Part model, mm, in its own coordinate system. Coordinates: 2 decimals unless noted, no trailing zeros. Loops run counter-clockwise (first coordinate to the right, second up) from the corner with the lowest first, then second, coordinate; pieces in that order, holes last. Notation, with made-up numbers: (-37, 30) - (3, 30) arc R28 cw to (3, 50) - close; hole circle Ø7 at (29.5, -26.5). An arc over 180 degrees is marked (long way). Answer as CSV lines item,"result".
from build123d import *

# Parameters (mm, degrees)
SKETCH_1_R                  = 17.5
SKETCH_1_R_2                = 11
EXTRUDE_1_DEPTH             = 2
HOLE_WIZARD_M3_1_AT_2_COUNT = 2
HOLE_WIZARD_M3_1_AT_2_PITCH = 20.152543264
HOLE_WIZARD_M3_1_AT_3_COUNT = 2
HOLE_WIZARD_M3_1_AT_3_PITCH = 28.5
HOLE_WIZARD_M3_1_AT_4_COUNT = 2
HOLE_WIZARD_M3_1_AT_4_PITCH = 20.152543264
HOLE_WIZARD_M3_1_AT_5_COUNT = 2
HOLE_WIZARD_M3_1_AT_5_PITCH = 14.25
CHAMFER_1_SIZE              = 0.25


with BuildPart() as part:
    # ｽｹｯﾁ1 → ﾎﾞｽ - 押し出し1 (new body)
    with BuildSketch(Plane.XY):
        Circle(SKETCH_1_R)
        Circle(SKETCH_1_R_2, mode=Mode.SUBTRACT)
    extrude(amount=EXTRUDE_1_DEPTH)

    # ｽｹｯﾁ4 → M3 丸皿ねじ用皿穴1 (revolve, cut)
    with BuildSketch(Plane(origin=(0, 14.25, 2), x_dir=(0, -1, 0), z_dir=(1, 0, 0))):
        Polygon((0, 0), (0, 2), (1.625, 2), (1.6, 1.975), (1.6, 1.55), (3.15, 0), align=None)
    hole_wizard_m3_1 = revolve(axis=Axis((0, 14.25, 8.35), (0, 0, -1)), mode=Mode.SUBTRACT)

    # M3 丸皿ねじ用皿穴1 at 2: M3 丸皿ねじ用皿穴1 ×2
    with Locations(*[Vector(0.7071067811865476, -0.7071067811865476, 0) * (i * HOLE_WIZARD_M3_1_AT_2_PITCH) for i in range(1, HOLE_WIZARD_M3_1_AT_2_COUNT)]):
        add(hole_wizard_m3_1, mode=Mode.SUBTRACT)

    # M3 丸皿ねじ用皿穴1 at 3: M3 丸皿ねじ用皿穴1 ×2
    with Locations(*[(0, -i * HOLE_WIZARD_M3_1_AT_3_PITCH, 0) for i in range(1, HOLE_WIZARD_M3_1_AT_3_COUNT)]):
        add(hole_wizard_m3_1, mode=Mode.SUBTRACT)

    # M3 丸皿ねじ用皿穴1 at 4: M3 丸皿ねじ用皿穴1 ×2
    with Locations(*[Vector(-0.7071067811865476, -0.7071067811865476, 0) * (i * HOLE_WIZARD_M3_1_AT_4_PITCH) for i in range(1, HOLE_WIZARD_M3_1_AT_4_COUNT)]):
        add(hole_wizard_m3_1, mode=Mode.SUBTRACT)

    # M3 丸皿ねじ用皿穴1 at 5: M3 丸皿ねじ用皿穴1 ×2
    with Locations(*[(0, -i * HOLE_WIZARD_M3_1_AT_5_PITCH, 0) for i in range(1, HOLE_WIZARD_M3_1_AT_5_COUNT)]):
        add(hole_wizard_m3_1, mode=Mode.SUBTRACT)

    # 面取り1
    # the kernel refuses this chamfer: 0.25 mm, written as the material it takes off along each edge
    with BuildSketch(Plane(origin=(0, 0, 2), x_dir=(1, 0, 0), z_dir=(0, -1, 0))) as chamfer_1_piece_1:
        Polygon((17.5, -CHAMFER_1_SIZE), (17.5 - CHAMFER_1_SIZE, 0), (17.5, 0), align=None)
    revolve(axis=Axis((0, 0, 2), (0, 0, 1)), mode=Mode.SUBTRACT)
    with BuildSketch(Plane(origin=(0, 0, 2), x_dir=(1, 0, 0), z_dir=(0, -1, 0))) as chamfer_1_piece_2:
        Polygon((11 + CHAMFER_1_SIZE, 0), (11, -CHAMFER_1_SIZE), (11, 0), align=None)
    revolve(axis=Axis((0, 0, 2), (0, 0, 1)), mode=Mode.SUBTRACT)


solid = part.part
Q1. Saw through at A-A (x = 0). Give the cut face in (y, z) (3 decimals), then the cut area to 3 significant figures.
Results:
outline,"(-17.5, 0) - (-15.875, 0) - (-15.85, 0.025) - (-15.85, 0.45) - (-17.325, 1.925) - (-17.5, 1.75) - close; (-12.65, 0.025) - (-12.625, 0) - (-11, 0) - (-11, 1.75) - (-11.175, 1.925) - (-12.65, 0.45) - close; (11, 0) - (12.625, 0) - (12.65, 0.025) - (12.65, 0.45) - (11.175, 1.925) - (11, 1.75) - close; (15.85, 0.025) - (15.875, 0) - (17.5, 0) - (17.5, 1.75) - (17.325, 1.925) - (15.85, 0.45) - close"
area,"8.29 mm^2"
Q2. Saw through at B-B (z = 1.15). Give the cut face in (x, y).
Results:
outline,"circle Ø35 at (0, 0); hole circle Ø4.6 at (-14.25, 0); hole circle Ø22 at (0, 0); hole circle Ø4.6 at (0, -14.25); hole circle Ø4.6 at (0, 14.25); hole circle Ø4.6 at (14.25, 0)"
Q3. Flat gauge pins, fed straight in: pin 1 (2 mm diameter, centred on x = 8, y = 1, fed in from +Z); pin 2 (1 mm diameter, centred on x = 9.5, z = 0.5, fed in from +Y); pin 3 (1 mm diameter, centred on x = 2, z = 1.5, fed in from -Y). Where does each tip first touch, or does it go through?
Results:
pin 1,"passes through"
pin 2,"stops at y = 15.01"
pin 3,"stops at y = -17.44"
Q4. Two-plate mould, pull along X, no slides. Class faces 1 (the face through (-8, -8, 0)), 2 (the face through (-0.07, -12.65, 0.24)): released by +X, released by -X, zero draft, split by the parting line, or undercut.
Results:
face 1,"zero draft"
face 2,"undercut"
Q5. Wall check: L1, parallel to Y at x = 0, z = 0.3; L2, parallel to Y at x = -3.5, z = 0.15; L3, parallel to Y at x = 0, z = 0.65. Give the ranges that are in metal, low to high.
Results:
L1,"y = -17.5 to -15.85, -12.65 to -11, 11 to 12.65, 15.85 to 17.5"
L2,"y = -17.15 to -10.43, 10.43 to 17.15"
L3,"y = -17.5 to -16.05, -12.45 to -11, 11 to 12.45, 16.05 to 17.5"
